Check sheet for the drawn part. Datum: minimum x, y, z corner. Units: mm. Give positions to 0.01 mm unless a question says otherwise; leave off trailing zeros. Loops run counter-clockwise (first coordinate to the right, second up) from the corner with the lowest first, then second, coordinate; pieces in that order, holes last.
1. Material ranges on L1, parallel to Z at x = 19.5, y = 12.5; L2, parallel to Z at x = 12, y = 15.5; L3, parallel to Y at x = 14, z = 10, recorded low to high.
2. Release check for a two-part mould opening along X. For the marked faces 1, 2 and 3 record: +X half, -X half, draft (parallel to the pull), parting line (faces both ways), or undercut.
3. Cross-section at B-B, the plane x = 2.25. Record the cut outline in (y, z) (3 decimals), plus the area to 3 significant figures.
4. Cross-section at D-D, the plane y = 14.25. Record the cut outline in (x, z) (3 decimals), plus the area to 3 significant figures.
5. Go/stop test with flat-tipped pins: pin 1 Ø10 at (y, z) = (7, 28) entering from -X; pin 2 Ø11 at (x, y) = (13, 14) entering from -Z; pin 3 Ø3 at (y, z) = (14.5, 1.5) entering from +X (3 decimals). Record where each tip stops, or that it passes through.
6. Cross-section at C-C, the plane z = 9.5. Record the cut outline in (x, y) (3 decimals), plus the area to 3 significant figures.
7. Cross-section at A-A, the plane y = 11.25. Record the cut outline in (x, z) (3 decimals), plus the area to 3 significant figures.
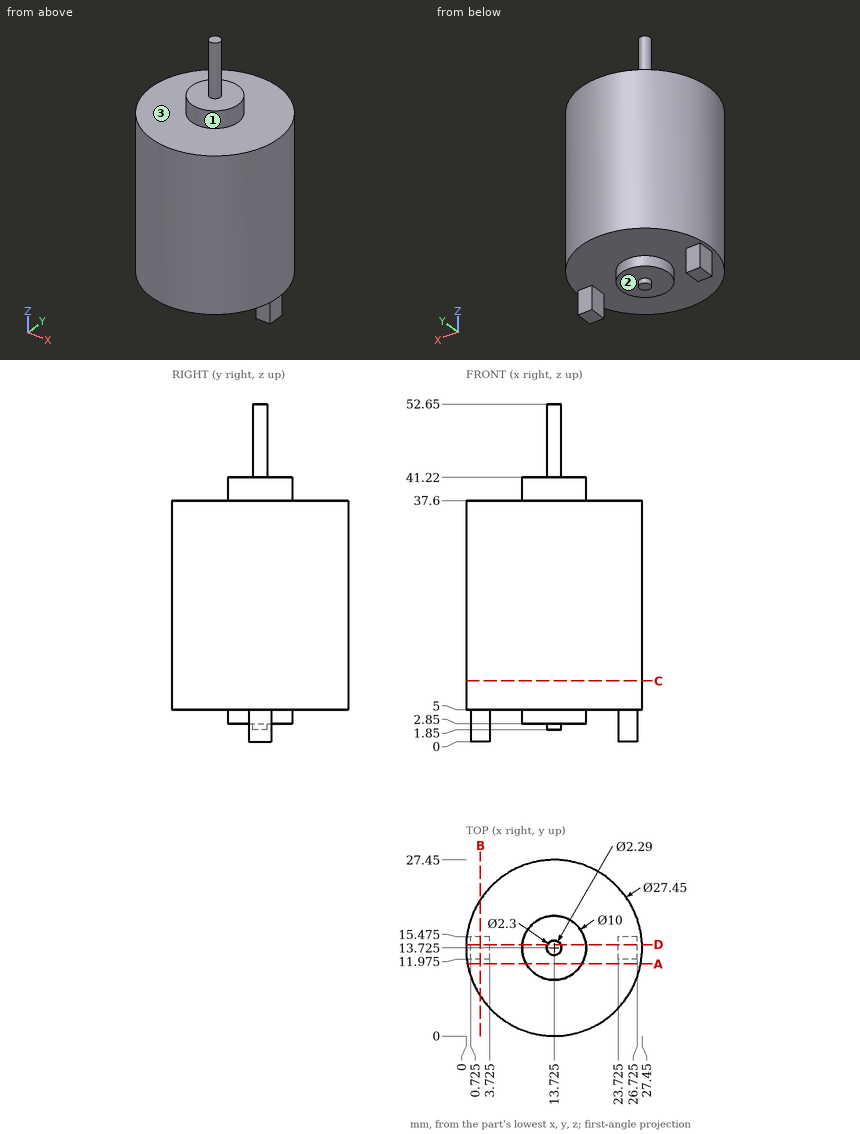
Result:
1. L1: z = 5 to 37.6
1. L2: z = 2.85 to 41.22
1. L3: y = 0 to 27.45
2. face 1: parting line
2. face 2: undercut
2. face 3: draft
3. outline: (6.195, 5) - (11.975, 5) - (11.975, 0) - (15.475, 0) - (15.475, 5) - (21.255, 5) - (21.255, 37.6) - (6.195, 37.6) - close
3. area: 508 mm2
4. outline: (0.01, 5) - (0.725, 5) - (0.725, 0) - (3.725, 0) - (3.725, 5) - (8.753, 5) - (8.753, 2.85) - (12.702, 2.85) - (12.702, 1.85) - (14.748, 1.85) - (14.748, 2.85) - (18.697, 2.85) - (18.697, 5) - (23.725, 5) - (23.725, 0) - (26.725, 0) - (26.725, 5) - (27.44, 5) - (27.44, 37.6) - (18.697, 37.6) - (18.697, 41.22) - (14.743, 41.22) - (14.743, 52.65) - (12.707, 52.65) - (12.707, 41.22) - (8.753, 41.22) - (8.753, 37.6) - (0.01, 37.6) - close
4. area: 1,010 mm2
5. pin 1: stops at x = 0.11
5. pin 2: stops at z = 1.85
5. pin 3: stops at x = 26.725
6. outline: circle Ø27.45 at (13.725, 13.725)
6. area: 592 mm2
7. outline: (0.225, 5) - (9.381, 5) - (9.381, 2.85) - (18.069, 2.85) - (18.069, 5) - (27.225, 5) - (27.225, 37.6) - (18.069, 37.6) - (18.069, 41.22) - (9.381, 41.22) - (9.381, 37.6) - (0.225, 37.6) - close
7. area: 930 mm2
